Verification items for the finished model (mm, model axes). Face numbers are marked on the shaded views. Round coordinates to 2 decimals unless told otherwise and drop trailing zeros. Write each loop counter-clockwise with the first axis right and the second up, starting at its lowest first coordinate (ties: lowest second). Pieces come first, ordered by that corner, then holes. Notation, with made-up numbers: M -13,40.25 L 41,40.25 A18 cw 41,53.25 Z; hole C 88,78 d4. An arc over 180 degrees is marked long. Answer in a Markdown table with one row per item. Add a question column.
1. Go/stop test with flat-tipped pins: pin 1 Ø1 at (y, z) = (1.5, -0.5) entering from -X; pin 2 Ø0.7 at (x, z) = (-62, 0.5) entering from +Y; pin 3 Ø1.2 at (x, z) = (58.5, 0.5) entering from +Y; pin 4 Ø5 at (x, y) = (41, 6) entering from +Z. Record where each tip stops, or that it passes through.
2. Sectioned sample at C-C on z = -5.75. Record the cut outline in (x, y), plus the area to 3 significant figures.
3. Draft check along X on the marked faces 1, 2, 3 and 4. Enter one of: pulls with the +X half, pulls with the -X half, needs draft (parallel to the pull), parting line crosses it, or undercut.
4. Material ranges on probe 1 along X at (y, z) = (9.5, 6.25); probe 2 along X at (y, z) = (7, 6); probe 3 along Y at (x, z) = (16, 2.25), recorded low to high.
5. Sectioned sample at A-A on y = 3. Record the cut outline in (x, z).
6. Sectioned sample at D-D on y = 11. Record the cut outline in (x, z), plus the area to 3 significant figures.
7. Sectioned sample at B-B on x = -35. Record the cut outline in (y, z).
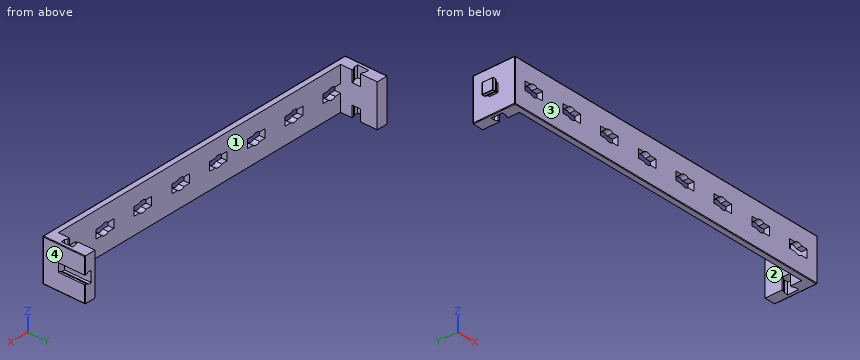
```python
from build123d import *

# Parameters (mm, degrees)
SKETCH_1_W                 = 120
SKETCH_1_H                 = 15
EXTRUDE_1_DEPTH            = 2
SKETCH_2_W                 = 4
SKETCH_2_H                 = 15
EXTRUDE_2_DEPTH            = 13
CUT_EXTRUDE_1_REACH        = 63.849
PATTERN_LINEAR_1_COUNT     = 5
PATTERN_LINEAR_1_PITCH     = 15
PATTERN_LINEAR_1_COL_COUNT = 4
PATTERN_LINEAR_1_COL_PITCH = 15
CUT_EXTRUDE_2_DEPTH        = 4
MIRROR_2_COPY_1_DEPTH      = 4
CUT_EXTRUDE_3_DEPTH        = 9.45
EXTRUDE_3_DEPTH            = 15
CUT_EXTRUDE_4_DEPTH        = 15
FILLET_1_R                 = 0.2
FILLET_2_R                 = 0.1


with BuildPart() as part:
    # 草图1 → 凸台-拉伸1 (new body)
    with BuildSketch(Plane(origin=(0, 0, 0), x_dir=(1, 0, 0), z_dir=(0, 1, 0))):
        Rectangle(SKETCH_1_W, SKETCH_1_H)
    extrude(amount=EXTRUDE_1_DEPTH)

    # 草图2 → 凸台-拉伸2 (add)
    with BuildSketch(Plane(origin=(0, 2, 0), x_dir=(1, 0, 0), z_dir=(0, 1, 0))):
        with Locations((-58, 0)):
            Rectangle(SKETCH_2_W, SKETCH_2_H)
        with Locations((58, 0)):
            Rectangle(SKETCH_2_W, SKETCH_2_H)
    extrude(amount=EXTRUDE_2_DEPTH)

    # 草图3 → 切除-拉伸1 (cut, up to next)
    with BuildSketch(Plane(origin=(0, 2, 0), x_dir=(1, 0, 0), z_dir=(0, 1, 0)), mode=Mode.PRIVATE) as cut_extrude_1_sk1:
        with BuildLine():
            Line((-4, -1.5), (-4, 1.5))
            Line((-4, 1.5), (-6.177124344, 1.5))
            ThreePointArc((-6.177124344, 1.5), (-7.5, 2), (-8.822875656, 1.5))
            Line((-8.822875656, 1.5), (-11, 1.5))
            Line((-11, 1.5), (-11, -1.5))
            Line((-11, -1.5), (-8.822875656, -1.5))
            ThreePointArc((-8.822875656, -1.5), (-7.5, -2), (-6.177124344, -1.5))
            Line((-6.177124344, -1.5), (-4, -1.5))
        make_face()
    cut_extrude_1_tool1 = extrude(cut_extrude_1_sk1.sketch, amount=-CUT_EXTRUDE_1_REACH, mode=Mode.PRIVATE) & part.part
    cut_extrude_1 = cut_extrude_1_tool1.solids().sort_by_distance((-7.5, 2, 0))[0]
    add(cut_extrude_1, mode=Mode.SUBTRACT)

    # 阵列(线性)1: 切除-拉伸1 ×5
    with Locations(*[(i * PATTERN_LINEAR_1_PITCH, 0, 0) for i in range(1, PATTERN_LINEAR_1_COUNT)]):
        add(cut_extrude_1, mode=Mode.SUBTRACT)

    # 阵列(线性)1 col: 切除-拉伸1 ×4
    with Locations(*[(-i * PATTERN_LINEAR_1_COL_PITCH, 0, 0) for i in range(1, PATTERN_LINEAR_1_COL_COUNT)]):
        add(cut_extrude_1, mode=Mode.SUBTRACT)

    # 草图4 → 切除-拉伸2 (cut)
    with BuildSketch(Plane.XY.offset(7.5)):
        with BuildLine():
            Line((-56, 6), (-56, 9))
            Line((-56, 9), (-56.677124344, 9))
            ThreePointArc((-56.677124344, 9), (-57.088161527, 9.280042303), (-57.555590279, 9.45))
            Line((-57.555590279, 9.45), (-58.8, 9.45))
            Line((-58.8, 9.45), (-58.8, 5.55))
            Line((-58.8, 5.55), (-57.555590279, 5.55))
            ThreePointArc((-57.555590279, 5.55), (-57.088161527, 5.719957697), (-56.677124344, 6))
            Line((-56.677124344, 6), (-56, 6))
        make_face()
    cut_extrude_2 = extrude(amount=-CUT_EXTRUDE_2_DEPTH, mode=Mode.SUBTRACT)

    # 镜向1: 切除-拉伸2 across plane
    add(cut_extrude_2.mirror(Plane.XY), mode=Mode.SUBTRACT)

    # 镜向2: 切除-拉伸2 across plane
    add(cut_extrude_2.mirror(Plane(origin=(0, 0, 0), x_dir=(0, 0, 1), z_dir=(1, 0, 0))), mode=Mode.SUBTRACT)

    # 镜向2 copy 1 sketch → 镜向2 copy 1 (cut)
    with BuildSketch(Plane(origin=(0, 0, -7.5), x_dir=(-1, 0, 0), z_dir=(0, 0, -1))):
        with BuildLine():
            Line((-56, 6), (-56, 9))
            Line((-56, 9), (-56.677124344, 9))
            ThreePointArc((-56.677124344, 9), (-57.088161527, 9.280042303), (-57.555590279, 9.45))
            Line((-57.555590279, 9.45), (-58.8, 9.45))
            Line((-58.8, 9.45), (-58.8, 5.55))
            Line((-58.8, 5.55), (-57.555590279, 5.55))
            ThreePointArc((-57.555590279, 5.55), (-57.088161527, 5.719957697), (-56.677124344, 6))
            Line((-56.677124344, 6), (-56, 6))
        make_face()
    extrude(amount=-MIRROR_2_COPY_1_DEPTH, mode=Mode.SUBTRACT)

    # 草图5 → 切除-拉伸3 (cut)
    with BuildSketch(Plane(origin=(0, 15, 0), x_dir=(1, 0, 0), z_dir=(0, 1, 0))):
        with BuildLine():
            Line((60, -1.5), (60, 1.5))
            Line((60, 1.5), (59.322875656, 1.5))
            ThreePointArc((59.322875656, 1.5), (58.911838473, 1.780042303), (58.444409721, 1.95))
            Line((58.444409721, 1.95), (57.5, 1.95))
            Line((57.5, 1.95), (57.5, -1.95))
            Line((57.5, -1.95), (58.444409721, -1.95))
            ThreePointArc((58.444409721, -1.95), (58.911838473, -1.780042303), (59.322875656, -1.5))
            Line((59.322875656, -1.5), (60, -1.5))
        make_face()
    extrude(amount=-CUT_EXTRUDE_3_DEPTH, mode=Mode.SUBTRACT)

    # 草图6 → 凸台-拉伸3 (add)
    with BuildSketch(Plane(origin=(0, 15, 0), x_dir=(1, 0, 0), z_dir=(0, 1, 0))):
        with BuildLine():
            Line((-60, -1.5), (-60, 1.5))
            Line((-60, 1.5), (-60.677124344, 1.5))
            ThreePointArc((-60.677124344, 1.5), (-61.088161527, 1.780042303), (-61.555590279, 1.95))
            Line((-61.555590279, 1.95), (-62.5, 1.95))
            Line((-62.5, 1.95), (-62.5, -1.95))
            Line((-62.5, -1.95), (-61.555590279, -1.95))
            ThreePointArc((-61.555590279, -1.95), (-61.088161527, -1.780042303), (-60.677124344, -1.5))
            Line((-60.677124344, -1.5), (-60, -1.5))
        make_face()
    extrude(amount=-EXTRUDE_3_DEPTH)

    # 草图7 → 切除-拉伸4 (cut)
    with BuildSketch(Plane.XY.offset(7.5)):
        with BuildLine():
            Line((-62.5, 9.45), (-61.555590279, 9.45))
            ThreePointArc((-61.555590279, 9.45), (-61.088161527, 9.280042303), (-60.677124344, 9))
            Line((-60.677124344, 9), (-60, 9))
            Line((-60, 9), (-60, 15))
            Line((-60, 15), (-62.5, 15))
            Line((-62.5, 15), (-62.5, 9.45))
        make_face()
        with BuildLine():
            Line((-60, 0), (-60, 6))
            Line((-60, 6), (-60.677124344, 6))
            ThreePointArc((-60.677124344, 6), (-61.088161527, 5.719957697), (-61.555590279, 5.55))
            Line((-61.555590279, 5.55), (-62.5, 5.55))
            Line((-62.5, 5.55), (-62.5, 0))
            Line((-62.5, 0), (-60, 0))
        make_face()
    extrude(amount=-CUT_EXTRUDE_4_DEPTH, mode=Mode.SUBTRACT)

    # 圆角1
    fillet_1_edges = [part.edges().sort_by_distance(p)[0] for p in [
        (-60, 15, 0),
        (60, 15, 4.5),
        (60, 15, -4.5),
        (60, 0, 0),
        (0, 0, 7.5),
        (-60, 0, 0),
        (0, 0, -7.5),
        (60, 7.5, -7.5),
        (60, 7.5, 7.5),
        (-60, 7.5, 7.5),
        (-60, 7.5, -7.5),
    ]]
    fillet(fillet_1_edges, radius=FILLET_1_R)

    # 圆角2
    fillet_2_edges = [part.edges().sort_by_distance(p)[0] for p in [
        (-62.5, 7.5, -1.95),
        (-62.5, 7.5, 1.95),
        (-62.5, 5.55, 0),
        (-62.5, 9.45, 0),
    ]]
    fillet(fillet_2_edges, radius=FILLET_2_R)


solid = part.part
```
Geometry check:
| question | item | result |
|---|---|---|
| 1 | pin 1 | stops at x = -60 |
| 1 | pin 2 | stops at y = 9.45 |
| 1 | pin 3 | stops at y = 5.55 |
| 1 | pin 4 | passes through |
| 2 | outline | M -60,0.2 A0.2 ccw -59.8,0 L 59.8,0 A0.2 ccw 60,0.2 L 60,14.8 A0.2 ccw 59.8,15 L 56,15 L 56,9 L 56.68,9 A2 cw 57.56,9.45 L 58.8,9.45 L 58.8,5.55 L 57.56,5.55 A2 cw 56.68,6 L 56,6 L 56,2 L -56,2 L -56,6 L -56.68,6 A2 cw -57.56,5.55 L -58.8,5.55 L -58.8,9.45 L -57.56,9.45 A2 cw -56.68,9 L -56,9 L -56,15 L -59.8,15 A0.2 ccw -60,14.8 Z |
| 2 | area | 324 mm2 |
| 3 | face 1 | undercut |
| 3 | face 2 | undercut |
| 3 | face 3 | needs draft |
| 3 | face 4 | pulls with the +X half |
| 4 | probe 1 | x = -60 to -56, 56 to 60 |
| 4 | probe 2 | x = -60 to -58.8, 58.8 to 60 |
| 4 | probe 3 | y = 0 to 2 |
| 5 | outline | M -60,-7.3 A0.2 ccw -59.8,-7.5 L -56,-7.5 L -56,7.5 L -59.8,7.5 A0.2 ccw -60,7.3 Z; M 56,-7.5 L 59.8,-7.5 A0.2 ccw 60,-7.3 L 60,7.3 A0.2 ccw 59.8,7.5 L 56,7.5 Z |
| 6 | outline | M -60,-7.3 A0.2 ccw -59.8,-7.5 L -56,-7.5 L -56,7.5 L -59.8,7.5 A0.2 ccw -60,7.3 Z; M 56,-7.5 L 59.8,-7.5 A0.2 ccw 60,-7.3 L 60,-1.5 L 59.32,-1.5 A2 cw 58.44,-1.95 L 57.5,-1.95 L 57.5,1.95 L 58.44,1.95 A2 cw 59.32,1.5 L 60,1.5 L 60,7.3 A0.2 ccw 59.8,7.5 L 56,7.5 Z |
| 6 | area | 111 mm2 |
| 7 | outline | M 0,-7.3 A0.2 ccw 0.2,-7.5 L 2,-7.5 L 2,-1.5 L 0,-1.5 Z; M 0,1.5 L 2,1.5 L 2,7.5 L 0.2,7.5 A0.2 ccw 0,7.3 Z |
